```python
from build123d import *

# Parameters (mm, degrees)
SKETCH_1_W      = 56
SKETCH_1_H      = 6
SKETCH_1_R      = 1.5
EXTRUDE_1_DEPTH = 4
FILLET_1_R      = 3
EXTRUDE_START   = 1
SKETCH_2_R      = 2.5
SKETCH_2_R_2    = 1.5
EXTRUDE_2_DEPTH = 1


with BuildPart() as part:
    # 草图1 → 凸台-拉伸1 (new body)
    with BuildSketch(Plane.XY):
        Rectangle(SKETCH_1_W, SKETCH_1_H)
        with Locations((-25, 0)):
            Circle(SKETCH_1_R, mode=Mode.SUBTRACT)
        with Locations((25, 0)):
            Circle(SKETCH_1_R, mode=Mode.SUBTRACT)
    extrude(amount=EXTRUDE_1_DEPTH)

    # 圆角1
    fillet_1_edges = [part.edges().sort_by_distance(p)[0] for p in [
        (28, -3, 2),
        (28, 3, 2),
        (-28, -3, 2),
        (-28, 3, 2),
    ]]
    fillet(fillet_1_edges, radius=FILLET_1_R - 0.0001)  # a hair under: the kernel refuses the full size

    # 草图2 → 凸台-拉伸2 (add)
    # profile 1 of 2: a face of its own
    with BuildSketch(Plane(origin=(0, 0, 0), x_dir=(-1, 0, 0), z_dir=(0, 0, -1)).offset(EXTRUDE_START)):
        with Locations((25, 0)):
            Circle(SKETCH_2_R)
        with Locations((25, 0)):
            Circle(SKETCH_2_R_2, mode=Mode.SUBTRACT)
    # profile 2 of 2: a face of its own
    with BuildSketch(Plane(origin=(0, 0, 0), x_dir=(-1, 0, 0), z_dir=(0, 0, -1)).offset(EXTRUDE_START)):
        with Locations((-25, 0)):
            Circle(SKETCH_2_R)
        with Locations((-25, 0)):
            Circle(SKETCH_2_R_2, mode=Mode.SUBTRACT)
    extrude(amount=-EXTRUDE_2_DEPTH)


solid = part.part
```
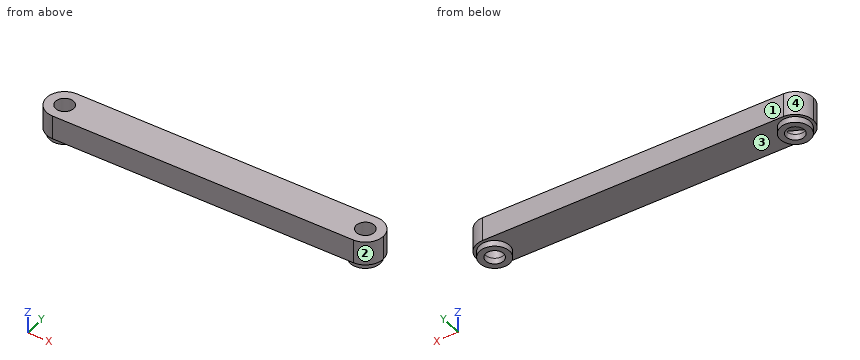
Read the model definition and answer for the solid it produces. Units are mm, in the model's axes. Face numbers are marked on the shaded views. Round coordinates to 2 decimals unless told otherwise and drop trailing zeros. Write each loop counter-clockwise with the first axis right and the second up, starting at its lowest first coordinate (ties: lowest second). Pieces come first, ordered by that corner, then holes. Notation, with made-up numbers: (59, -19) -> (108, -19) arc R15 ccw to (108, 3) -> close; hole circle Ø1 at (-39.5, 33.25). An arc over 180 degrees is marked (long way). Answer in a Markdown table with one row per item. Add a question column.
1) Given P1, Ø3, axis at x = -12, y = -1, coming from the -Z side, flat-ended and moving along its own axis, determine where the tip first touches the part or whether it passes through.
2) Determine the mould class of the marked faces 1, 2, 3 and 4 for opening direction X: pulls with the +X half, pulls with the -X half, needs draft (parallel to the pull), parting line crosses it, or undercut.
3) Find section C-C, the plane x = -10. Determine the outline of the cut face in (y, z), and give its area (3 significant figures).
4) Find section A-A, the plane z = 0.85. State how many separate pieces and enclosed holes the cut face has, and give its area (3 significant figures).
5) Consider line 1 (X direction, y = 0, z = 2.7); line 2 (Y direction, x = 25, z = -0.75); line 3 (X direction, y = -1.25, z = 3.25). Determine where each line is inside the solid, lowest interval first.
Findings below:
| question | item | result |
|---|---|---|
| 1 | P1 | z = 0 |
| 2 | face 1 | needs draft |
| 2 | face 2 | pulls with the +X half |
| 2 | face 3 | undercut |
| 2 | face 4 | pulls with the -X half |
| 3 | outline | (-3, 0) -> (3, 0) -> (3, 4) -> (-3, 4) -> close |
| 3 | area | 24.0 mm² |
| 4 | separate pieces | 1 |
| 4 | enclosed holes | 2 |
| 4 | area | 314 mm² |
| 5 | line 1 | -28 to -26.5, -23.5 to 23.5, 26.5 to 28 |
| 5 | line 2 | -2.5 to -1.5, 1.5 to 2.5 |
| 5 | line 3 | -27.73 to -25.83, -24.17 to 24.17, 25.83 to 27.73 |
